Could you check a few things on this model? Use its own coordinates, in mm. A direction names the side the tool comes from. Coordinates: 2 decimals unless noted, no trailing zeros. Order: outer loops, then holes, each group sorted by start corner. A loop starts at its lowest first (then second) coordinate and runs counter-clockwise, first axis right, second up. Notation, with made-up numbers: (-23, 43.5) - (23, 43.5) arc R17 ccw to (23, 54.5) - close; hole circle Ø6 at (20, 85.25). An arc over 180 degrees is marked (long way). One line per item, written item: value.
from build123d import *

# Parameters (mm, degrees)
SKETCH005_W          = 180
SKETCH005_H          = 132
SKETCH003_W          = 176
SKETCH003_H          = 132
SKETCH004_W          = 180
SKETCH004_H          = 132
SKETCH_W             = 10
SKETCH_H             = 4
POCKET_DEPTH         = 2.001
POCKET_DEPTH_BACK    = 2.001
SKETCH001_W          = 10
SKETCH001_H          = 4
POCKET001_DEPTH      = 2.001
POCKET001_DEPTH_BACK = 2.001
SKETCH002_W          = 10
SKETCH002_H          = 4
POCKET002_DEPTH      = 2.001
POCKET002_DEPTH_BACK = 2.001
POCKET003_DEPTH      = 128.001
POCKET003_DEPTH_BACK = 4.001
POCKET004_DEPTH      = 128.001
POCKET004_DEPTH_BACK = 4.001
POCKET005_DEPTH      = 128.001
POCKET005_DEPTH_BACK = 4.001
FILLET_R             = 1
POCKET006_DEPTH      = 2.001
POCKET006_DEPTH_BACK = 2.001


with BuildPart() as part:
    # Sketch005 (on DatumPlane) → AdditiveLoft section 0
    with BuildSketch(Plane.XY.offset(-2)):
        with Locations((0, 62)):
            Rectangle(SKETCH005_W, SKETCH005_H)
    # Sketch003 → AdditiveLoft section 1
    with BuildSketch(Plane.XY):
        with Locations((0, 62)):
            Rectangle(SKETCH003_W, SKETCH003_H)
    # Sketch004 (on DatumPlane) → AdditiveLoft section 2
    with BuildSketch(Plane.XY.offset(2)):
        with Locations((0, 62)):
            Rectangle(SKETCH004_W, SKETCH004_H)
    loft(ruled=True)

    # Sketch → Pocket (cut, two sides)
    with BuildSketch(Plane.XY) as pocket_sk:
        with Locations((-75, 2)):
            Rectangle(SKETCH_W, SKETCH_H)
        with Locations((0, 2)):
            Rectangle(SKETCH_W, SKETCH_H)
        with Locations((75, 2)):
            Rectangle(SKETCH_W, SKETCH_H)
    extrude(amount=-POCKET_DEPTH, mode=Mode.SUBTRACT)
    extrude(pocket_sk.sketch, amount=POCKET_DEPTH_BACK, mode=Mode.SUBTRACT)

    # Sketch001 (on DatumPlane) → Pocket001 (cut, two sides)
    with BuildSketch(Plane(origin=(0, 60, 0), x_dir=(1, 0, 0), z_dir=(0, 0, 1))) as pocket001_sk:
        with Locations((-75, 2)):
            Rectangle(SKETCH001_W, SKETCH001_H)
        with Locations((0, 2)):
            Rectangle(SKETCH001_W, SKETCH001_H)
        with Locations((75, 2)):
            Rectangle(SKETCH001_W, SKETCH001_H)
    extrude(amount=-POCKET001_DEPTH, mode=Mode.SUBTRACT)
    extrude(pocket001_sk.sketch, amount=POCKET001_DEPTH_BACK, mode=Mode.SUBTRACT)

    # Sketch002 (on DatumPlane) → Pocket002 (cut, two sides)
    with BuildSketch(Plane(origin=(0, 124, 0), x_dir=(1, 0, 0), z_dir=(0, 0, 1))) as pocket002_sk:
        with Locations((-75, 2)):
            Rectangle(SKETCH002_W, SKETCH002_H)
        with Locations((0, 2)):
            Rectangle(SKETCH002_W, SKETCH002_H)
        with Locations((75, 2)):
            Rectangle(SKETCH002_W, SKETCH002_H)
    extrude(amount=-POCKET002_DEPTH, mode=Mode.SUBTRACT)
    extrude(pocket002_sk.sketch, amount=POCKET002_DEPTH_BACK, mode=Mode.SUBTRACT)

    # Sketch006 → Pocket003 (cut, two sides)
    with BuildSketch(Plane.XZ) as pocket003_sk:
        Polygon((-11.5, 0), (-7.5, 0), (-8.5, 2), (-10.5, 2), align=None)
        Polygon((7.5, 0), (11.5, 0), (10.5, 2), (8.5, 2), align=None)
    extrude(amount=-POCKET003_DEPTH, mode=Mode.SUBTRACT)
    extrude(pocket003_sk.sketch, amount=POCKET003_DEPTH_BACK, mode=Mode.SUBTRACT)

    # Sketch007 (on DatumPlane) → Pocket004 (cut, two sides)
    with BuildSketch(Plane(origin=(-75, 0, 0), x_dir=(1, 0, 0), z_dir=(0, -1, 0))) as pocket004_sk:
        Polygon((-11.5, 0), (-7.5, 0), (-8.5, 2), (-10.5, 2), align=None)
        Polygon((7.5, 0), (11.5, 0), (10.5, 2), (8.5, 2), align=None)
    extrude(amount=-POCKET004_DEPTH, mode=Mode.SUBTRACT)
    extrude(pocket004_sk.sketch, amount=POCKET004_DEPTH_BACK, mode=Mode.SUBTRACT)

    # Sketch008 (on DatumPlane) → Pocket005 (cut, two sides)
    with BuildSketch(Plane(origin=(75, 0, 0), x_dir=(1, 0, 0), z_dir=(0, -1, 0))) as pocket005_sk:
        Polygon((-11.5, 0), (-7.5, 0), (-8.5, 2), (-10.5, 2), align=None)
        Polygon((7.5, 0), (11.5, 0), (10.5, 2), (8.5, 2), align=None)
    extrude(amount=-POCKET005_DEPTH, mode=Mode.SUBTRACT)
    extrude(pocket005_sk.sketch, amount=POCKET005_DEPTH_BACK, mode=Mode.SUBTRACT)

    # Fillet
    fillet_edges = [part.edges().sort_by_distance(p)[0] for p in [
        (-70, 2, -2),
        (-80, 2, -2),
        (-5, 2, -2),
        (5, 2, -2),
        (70, 2, -2),
        (80, 2, -2),
        (-80, 62, -2),
        (-70, 62, -2),
        (-5, 62, -2),
        (5, 62, -2),
        (70, 62, -2),
        (80, 62, -2),
        (-80, 126, -2),
        (-70, 126, -2),
        (-5, 126, -2),
        (5, 126, -2),
        (70, 126, -2),
        (80, 126, -2),
    ]]
    fillet(fillet_edges, radius=FILLET_R)

    # Sketch009 → Pocket006 (cut, two sides)
    with BuildSketch(Plane.XY) as pocket006_sk:
        Polygon((-100, 0), (-100, -20), (100, -20), (100, 0), (87.5, 0), (82.5, -4), (67.5, -4), (62.5, 0), (12.5, 0), (7.5, -4), (-7.5, -4), (-12.5, 0), (-62.5, 0), (-67.5, -4), (-82.5, -4), (-87.5, 0), align=None)
    extrude(amount=-POCKET006_DEPTH, mode=Mode.SUBTRACT)
    extrude(pocket006_sk.sketch, amount=POCKET006_DEPTH_BACK, mode=Mode.SUBTRACT)


solid = part.part
Item 1: I'm going to push flat-ended pins straight in: pin 1 Ø1 at (y, z) = (99, 1) entering from +X; pin 2 Ø1.2 at (x, z) = (74, -0.5) entering from +Y; pin 3 Ø0.9 at (y, z) = (126.5, 0) entering from -X. Where does each tip first touch, or does it pass through?
Conclusion:
pin 1: x = 89.5
pin 2: y = 124
pin 3: x = -88.45
Item 2: If I drill on probe 1 along Y at (x, z) = (72, -1.2); probe 2 along Y at (x, z) = (-50, -0.1); probe 3 along X at (y, z) = (57.5, -1.8), over which ranges is the centre line in solid material (lowest first)?
Conclusion:
probe 1: -4 to 0, 4 to 60, 64 to 124
probe 2: 0 to 128
probe 3: -89.8 to 89.8
Item 3: I want a section at C-C on x = 23. Please give me the cut outline in (y, z).
Conclusion:
outline: (0, -2) - (128, -2) - (128, 2) - (0, 2) - close
Item 4: I want a section at B-B on z = 0.8. Give the number of separate pieces and of enclosed holes in the cut face, then the cut area to 3 significant figures.
Conclusion:
separate pieces: 7
enclosed holes: 6
area: 20,100 mm²
Item 5: For faces 4 (the face through (38, 0, 0)), 5 (the face through (38, 128, 0)), which set-ups out of +Z, -Z, +X, -X, +Y, -Y let a thin tool reach every point of the face, with its end or its side?
Conclusion:
face 4: +Z, -Z, -Y
face 5: +Z, -Z, +X, -X, +Y
Item 6: Thinking about a two-plate mould opening in Y: for faces 1 (the face through (-75, 60, 0)), 2 (the face through (-39, 63, 2)), 3 (the face through (0, -4, 0)), which applies, pulls with the +Y half, pulls with the -Y half, needs draft (parallel to the pull), parting line crosses it, or undercut?
Conclusion:
face 1: undercut
face 2: needs draft
face 3: pulls with the -Y half
